Model file for the job. Use its own axes, mm. A direction names the side the tool comes from. Round coordinates to 2 decimals unless told otherwise and drop trailing zeros. Order: outer loops, then holes, each group sorted by start corner. A loop starts at its lowest first (then second) coordinate and runs counter-clockwise, first axis right, second up. Notation, with made-up numbers: (47, 51.25) - (51, 51.25) arc R20 cw to (51, 75.25) - close; hole circle Ø7 at (65.25, -19.5). An arc over 180 degrees is marked (long way). Answer as CSV lines item,"result". Start each with the question number.
1. Pin check, flat tips, straight feed: pin 1 Ø5 at (x, y) = (-1.5, -20) entering from +Z; pin 2 Ø8 at (x, y) = (29.5, -36.5) entering from +Z; pin 3 Ø5 at (x, y) = (49.5, -27.5) entering from -Z; pin 4 Ø2 at (x, z) = (-89.5, -52) entering from +Y. Stop position of each tip, or through.
2. Pull direction Z, two halves, no side cores. Call faces 4 (the face through (104.92, -24.58, -33.04)), 5 (the face through (73, -55, 83)), 6 (the face through (109.69, -25.09, -34.54)): released by +Z, released by -Z, zero draft, split by the parting line, or undercut.
3. 3-axis set-ups, long thin cutter, end or side, ignore diameter. For faces 1 (the face through (110.34, -17.01, 0.84)), 2 (the face through (97.3, 5, -40.2)), 3 (the face through (16.058, -20.396, 110.989)): which of +Z, -Z, +X, -X, +Y, -Y reach the whole face in a straight line?
4. Band-saw the part on C-C on y = -42.5. List the corners of the cut face in (x, z).
5. Wall check: line 1 along Z through (x, y) = (0, -8); line 2 along X through (y, z) = (6.9, 0). Give the ranges that are in metal, low to high. Write a range as [from, to].
6. Band-saw the part on D-D on y = -2.5. List the corners of the cut face in (x, z).
7. Band-saw the part on B-B on z = 0. List the corners of the cut face in (x, y), then the cut area to 3 significant figures.
8. Band-saw the part on A-A on x = 0. List the corners of the cut face in (y, z).
Autodesk Inventor part; units mm, degrees
ref_plane "YZ Plane" through (0, 0, 0) normal (1, 0, 0) x (0, 1, 0)
ref_plane "XZ Plane" through (0, 0, 0) normal (0, 1, 0) x (-1, 0, 0)
ref_plane "XY Plane" through (0, 0, 0) normal (0, 0, 1) x (1, 0, 0)
sketch "草圖1" plane through (0, 0, 0) normal (0, 1, 0) x (-1, 0, 0)
  circle A0 centre (0, 0) radius 110
  dimension "d0" = 220
extrude "擠出1" add sketch "草圖1" along normal blind 4
sketch "草圖2" plane through (0, 4, 0) normal (0, 1, 0) x (1, 0, 0)
  circle A0 centre (0, 0) radius 110
sketch "草圖3" plane through (0, 4, 0) normal (0, 1, 0) x (1, 0, 0)
  circle A0 centre (0, 0) radius 110
  circle A1 centre (0, 0) radius 115
  circle A2 centre (0, 0) radius 105
  dimension "d3" = 5
  dimension "d4" = 5
extrude "擠出2" add sketch "草圖3" against normal blind 59 contours A1
sketch "草圖4" plane through (0, 4, 0) normal (0, 1, 0) x (1, 0, 0)
  circle A0 centre (0, 0) radius 115
  circle A1 centre (0, 0) radius 110
  circle A2 centre (0, 0) radius 105
  dimension "d7" = 5
extrude "擠出3" add sketch "草圖4" along normal blind 5 contours A0 | A1
sketch "草圖5" plane through (0, 0, 0) normal (0, -1, 0) x (1, 0, 0)
  circle A0 centre (0, 0) radius 110
  circle A1 centre (0, 0) radius 110
  dimension "d10" = 220
extrude "擠出4" cut sketch "草圖5" against normal blind 5
fillet "圓角2" radius 5 1 edges at (-115, 9, 0)
sketch "草圖6" plane through (0, 0, 0) normal (0, 0, 1) x (1, 0, 0)
  line L0 (-115, -55) -> (115, -55)
  line L1 (0, -53) -> (25, -53)
  line L2 (0, -53) -> (-25, -53)
  line L3 (-25, -53) -> (-25, -32)
  line L4 (25, -53) -> (25, -32)
  line L5 (-25, -32) -> (-13, -32)
  circle A0 centre (-13, -32) radius 8.1
  arc A1 (-2.7801, -25.7108) -> (-25, -32) centre (-13, -32) ccw
  circle A2 centre (13, -32) radius 8.1
  arc A3 (25, -32) -> (2.7801, -25.7108) centre (13, -32) ccw
  arc A4 (-2.7801, -25.7108) -> (2.7801, -25.7108) centre (0, -24) ccw
  line L6 (0, -55) -> (-25, -55)
  line L7 (-25, -55) -> (-25, -53)
  line L8 (0, -55) -> (25, -55)
  line L9 (25, -53) -> (25, -55)
  point P0 (0, 0)
  dimension "d15" = 25
  dimension "d16" = 25
  dimension "d17" = 21
  dimension "d18" = 21
  dimension "d19" = 12
  dimension "d20" = 16.2
  dimension "d22" = 25
  dimension "d23" = 2
extrude "擠出5" cut sketch "草圖6" along normal blind 200 contours L7 L2 L1 L9 L0 | A0 | L3 A1 A4 A3 L4 L1 L2 | A2
sketch "草圖7" plane through (0, 0, 0) normal (1, 0, 0) x (0, 1, 0)
  line L0 (-55, 112.2497) -> (-55, -115)
  line L1 (-55, 0) -> (-55, -38)
  line L2 (-55, 0) -> (-55, 38)
  circle A0 centre (-55, 0) radius 38
  point P0 (0, 0)
  dimension "d26" = 38
  dimension "d27" = 38
extrude "擠出6" cut sketch "草圖7" along normal mid plane 400 contours A0 L0 picked at (-29.9842, -2.8186)
properties part number "Shell-disc"
Reply:
1,pin 1,"stops at z = 115"
1,pin 2,"stops at z = 112.14"
1,pin 3,"stops at z = -104.96"
1,pin 4,"passes through"
2,face 4,"undercut"
2,face 5,"zero draft"
2,face 6,"split by the parting line"
3,face 1,"+X, -X, -Y"
3,face 2,"-Y"
3,face 3,"+Z, -Y"
4,outline,"(-109.26, -35.89) arc R115 ccw to (109.26, -35.89) - (103.98, -35.89) arc R110 cw to (-103.98, -35.89) - close; (-109.26, 35.89) - (-103.98, 35.89) arc R110 cw to (-25, 107.12) - (-25, 112.25) arc R115 ccw to start; (25, 107.12) arc R110 cw to (103.98, 35.89) - (109.26, 35.89) arc R115 ccw to (25, 112.25) - close"
5,line 1,"z = [-115, -110], [110, 115]"
5,line 2,"x = [-114.07, -105], [105, 114.07]"
6,outline,"circle Ø230 at (0, 0); hole circle Ø220 at (0, 0)"
7,outline,"(-115, -17) - (-110, -17) - (-110, 5) - (-105, 5) - (-105, 9) - (-110, 9) arc R5 ccw to (-115, 4) - close; (105, 5) - (110, 5) - (110, -17) - (115, -17) - (115, 4) arc R5 ccw to (110, 9) - (105, 9) - close"
7,area,"289 mm2"
8,outline,"(-55, -115) - (4, -115) arc R5 ccw to (9, -110) - (9, -105) - (5, -105) - (5, -110) - (-55, -110) - close; (-27.26, 110) - (5, 110) - (5, 105) - (9, 105) - (9, 110) arc R5 ccw to (4, 115) - (-27.26, 115) - close"
